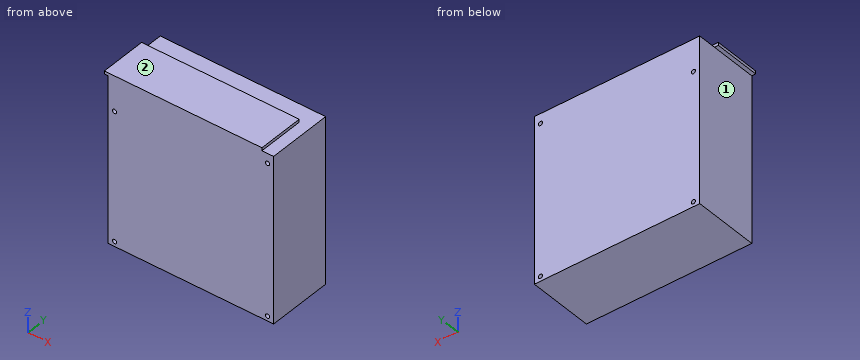
from build123d import *

# Parameters (mm, degrees)
SKETCH1_W            = 170
SKETCH1_H            = 170
BOSS_EXTRUDE1_DEPTH  = 67
SKETCH2_W            = 162
SKETCH2_H            = 48
BOSS_EXTRUDE2_DEPTH  = 3
M4_CLEARANCE_HOLE1_D = 4.3


with BuildPart() as part:
    # Sketch1 → Boss-Extrude1 (new body)
    with BuildSketch(Plane(origin=(0, 0, 0), x_dir=(1, 0, 0), z_dir=(0, 1, 0))):
        Rectangle(SKETCH1_W, SKETCH1_H)
    extrude(amount=BOSS_EXTRUDE1_DEPTH)

    # Sketch2 → Boss-Extrude2 (add)
    with BuildSketch(Plane.XY.offset(85)):
        with Locations((-8, 24)):
            Rectangle(SKETCH2_W, SKETCH2_H)
    extrude(amount=BOSS_EXTRUDE2_DEPTH)

    # M4 Clearance Hole1 (through all)
    with Locations(Plane(origin=(0, 67, 0), x_dir=(1, 0, 0), z_dir=(0, 1, 0))):
        with Locations((-78.5, 80), (-78.5, -52), (78.75, -75), (78.75, 80)):
            Hole(M4_CLEARANCE_HOLE1_D / 2)


solid = part.part
Read the model definition and answer for the solid it produces. Units are mm, in the model's axes. Face numbers are marked on the shaded views. A direction names the side the tool comes from. Round coordinates to 2 decimals unless told otherwise and drop trailing zeros. Write each loop counter-clockwise with the first axis right and the second up, starting at its lowest first coordinate (ties: lowest second). Pieces come first, ordered by that corner, then holes. Notation, with made-up numbers: (44.25, 23) - (100.25, 23) arc R21 cw to (100.25, 42) - close; hole circle Ø6 at (54.5, 47.25). An arc over 180 degrees is marked (long way). Use a Markdown table: item, result.
(1) Straight lines are drawn through the part: line 1 along X through (y, z) = (28, -80); line 2 along Z through (x, y) = (-78.5, 39); line 3 along X through (y, z) = (21.5, 75). For each, find the intervals that lie inside material, in ascending order. Write a range as [from, to].
Reported:
| item | result |
|---|---|
| line 1 | [-85, -80.65], [-76.35, 76.6], [80.9, 85] |
| line 2 | [-85, -82.15], [-77.85, 49.85], [54.15, 88] |
| line 3 | [-85, 76.6], [80.9, 85] |
(2) Which of the six approach directions +Z, -Z, +X, -X, +Y, -Y give full straight-line access (tool end or side, diameter ignored) to the marked faces 1 and 2?
Reported:
| item | result |
|---|---|
| face 1 | -Z, -X, +Y, -Y |
| face 2 | +Z, +X, -X, +Y, -Y |
(3) Each of these flat-tipped pins is pushed along its axis until it touches: pin 1 Ø4 at (x, z) = (-78.5, 52) entering from -Y; pin 2 Ø6 at (x, y) = (5.5, 59.5) entering from +Z; pin 3 Ø1.5 at (y, z) = (49.5, -1) entering from -X; pin 4 Ø2.5 at (y, z) = (20.5, 87) entering from +X. Where does it stop, or does it pass through?
Reported:
| item | result |
|---|---|
| pin 1 | through |
| pin 2 | z = 85 |
| pin 3 | x = -85 |
| pin 4 | x = 73 |
(4) The part is cut by section B-B (x = -78.5). Write down the section's boundary in (y, z).
Reported:
| item | result |
|---|---|
| outline | (0, -85) - (67, -85) - (67, -82.15) - (0, -82.15) - close; (0, -77.85) - (67, -77.85) - (67, 49.85) - (0, 49.85) - close; (0, 54.15) - (67, 54.15) - (67, 85) - (48, 85) - (48, 88) - (0, 88) - close |
(5) The part is cut by section A-A (z = -80). Write down the section's boundary in (x, y).
Reported:
| item | result |
|---|---|
| outline | (-85, 0) - (-80.65, 0) - (-80.65, 67) - (-85, 67) - close; (-76.35, 0) - (76.6, 0) - (76.6, 67) - (-76.35, 67) - close; (80.9, 0) - (85, 0) - (85, 67) - (80.9, 67) - close |
(6) The part is cut by section C-C (y = 54). Write down the section's boundary in (x, z), then the cut area to 3 significant figures.
Reported:
| item | result |
|---|---|
| outline | (-85, -85) - (85, -85) - (85, 85) - (-85, 85) - close; hole circle Ø4.3 at (-78.5, -80); hole circle Ø4.3 at (-78.5, 52); hole circle Ø4.3 at (78.75, -80); hole circle Ø4.3 at (78.75, 75) |
| area | 28,800 mm2 |
(7) The part is cut by section D-D (z = 75). Write down the section's boundary in (x, y).
Reported:
| item | result |
|---|---|
| outline | (-85, 0) - (76.6, 0) - (76.6, 67) - (-85, 67) - close; (80.9, 0) - (85, 0) - (85, 67) - (80.9, 67) - close |
